Verification items for the finished model (mm, model axes). Face numbers are marked on the shaded views. A direction names the side the tool comes from. Round coordinates to 2 decimals unless told otherwise and drop trailing zeros. Order: outer loops, then holes, each group sorted by start corner. A loop starts at its lowest first (then second) coordinate and runs counter-clockwise, first axis right, second up. Notation, with made-up numbers: M -13,84.25 L 14,84.25 A35 ccw 14,119.25 Z; hole C -30,-21 d11. An arc over 180 degrees is marked long. Write item = value, one per line. Start each with the question number.
from build123d import *

# Parameters (mm, degrees)
SKETCH_1_W          = 35
SKETCH_1_H          = 53
EXTRUDE_1_DEPTH     = 2
SKETCH_2_W          = 2
SKETCH_2_H          = 53
EXTRUDE_2_DEPTH     = 13.2
SKETCH_3_W          = 31
SKETCH_3_H          = 3
EXTRUDE_3_DEPTH     = 7.2
SKETCH_4_W          = 31
SKETCH_4_H          = 3
EXTRUDE_4_DEPTH     = 13.2
CUT_EXTRUDE_1_REACH = 57.956
SKETCH_5_R          = 1.25
SKETCH_7_W          = 31
SKETCH_7_H          = 3
CUT_EXTRUDE_2_DEPTH = 2.2
SKETCH_8_W          = 31
SKETCH_8_H          = 3
CUT_EXTRUDE_3_DEPTH = 2
SKETCH_10_W         = 11
SKETCH_10_H         = 3
CUT_EXTRUDE_4_DEPTH = 4
CUT_EXTRUDE_START   = -3
SKETCH_9_R          = 1.25
CUT_EXTRUDE_5_DEPTH = 3
SKETCH_12_W         = 2
SKETCH_12_H         = 10
CUT_EXTRUDE_6_DEPTH = 4
SKETCH_13_W         = 33
SKETCH_13_H         = 47
CUT_EXTRUDE_7_DEPTH = 4


with BuildPart() as part:
    # 草图1 → 凸台-拉伸1 (new body)
    with BuildSketch(Plane.XY):
        with Locations((2.5, -6.5)):
            Rectangle(SKETCH_1_W, SKETCH_1_H)
    extrude(amount=EXTRUDE_1_DEPTH)

    # 草图2 → 凸台-拉伸2 (add)
    with BuildSketch(Plane.XY.offset(2)):
        with Locations((-14, -6.5)):
            Rectangle(SKETCH_2_W, SKETCH_2_H)
        with Locations((19, -6.5)):
            Rectangle(SKETCH_2_W, SKETCH_2_H)
    extrude(amount=EXTRUDE_2_DEPTH)

    # 草图3 → 凸台-拉伸3 (add)
    with BuildSketch(Plane.XY.offset(2)):
        with Locations((2.5, 18.5)):
            Rectangle(SKETCH_3_W, SKETCH_3_H)
        with Locations((2.5, -31.5)):
            Rectangle(SKETCH_3_W, SKETCH_3_H)
    extrude(amount=EXTRUDE_3_DEPTH)

    # 草图4 → 凸台-拉伸4 (add)
    with BuildSketch(Plane.XY.offset(2)):
        with Locations((2.5, 15.5)):
            Rectangle(SKETCH_4_W, SKETCH_4_H)
        with Locations((2.5, -28.5)):
            Rectangle(SKETCH_4_W, SKETCH_4_H)
    extrude(amount=EXTRUDE_4_DEPTH)

    # 草图5 → 切除-拉伸1 (cut, up to next)
    with BuildSketch(Plane(origin=(0, 17, 0), x_dir=(1, 0, 0), z_dir=(0, 1, 0)), mode=Mode.PRIVATE) as cut_extrude_1_sk1:
        with Locations(Location((-8, -11.2, 0), (0, 0, 270))):
            Circle(SKETCH_5_R)
    cut_extrude_1_tool1 = extrude(cut_extrude_1_sk1.sketch, amount=-CUT_EXTRUDE_1_REACH, mode=Mode.PRIVATE) & part.part
    # 草图5 → 切除-拉伸1 (cut, up to next)
    with BuildSketch(Plane(origin=(0, 17, 0), x_dir=(1, 0, 0), z_dir=(0, 1, 0)), mode=Mode.PRIVATE) as cut_extrude_1_sk2:
        with Locations(Location((2.5, -11.2, 0), (0, 0, 270))):
            Circle(SKETCH_5_R)
    cut_extrude_1_tool2 = extrude(cut_extrude_1_sk2.sketch, amount=-CUT_EXTRUDE_1_REACH, mode=Mode.PRIVATE) & part.part
    # 草图5 → 切除-拉伸1 (cut, up to next)
    with BuildSketch(Plane(origin=(0, 17, 0), x_dir=(1, 0, 0), z_dir=(0, 1, 0)), mode=Mode.PRIVATE) as cut_extrude_1_sk3:
        with Locations(Location((13, -11.2, 0), (0, 0, 270))):
            Circle(SKETCH_5_R)
    cut_extrude_1_tool3 = extrude(cut_extrude_1_sk3.sketch, amount=-CUT_EXTRUDE_1_REACH, mode=Mode.PRIVATE) & part.part
    add(cut_extrude_1_tool1.solids().sort_by_distance((-8, 17, 11.2))[0], mode=Mode.SUBTRACT)
    add(cut_extrude_1_tool2.solids().sort_by_distance((2.5, 17, 11.2))[0], mode=Mode.SUBTRACT)
    add(cut_extrude_1_tool3.solids().sort_by_distance((13, 17, 11.2))[0], mode=Mode.SUBTRACT)

    # 草图7 → 切除-拉伸2 (cut)
    with BuildSketch(Plane.XY.offset(15.2)):
        with Locations((2.5, 15.5)):
            Rectangle(SKETCH_7_W, SKETCH_7_H)
    extrude(amount=-CUT_EXTRUDE_2_DEPTH, mode=Mode.SUBTRACT)

    # 草图8 → 切除-拉伸3 (cut)
    with BuildSketch(Plane.XY.offset(15.2)):
        with Locations((2.5, -28.5)):
            Rectangle(SKETCH_8_W, SKETCH_8_H)
    extrude(amount=-CUT_EXTRUDE_3_DEPTH, mode=Mode.SUBTRACT)

    # 草图10 → 切除-拉伸4 (cut)
    with BuildSketch(Plane.XY.offset(13.2)):
        with Locations((2.5, -28.5)):
            Rectangle(SKETCH_10_W, SKETCH_10_H)
    extrude(amount=-CUT_EXTRUDE_4_DEPTH, mode=Mode.SUBTRACT)

    # 草图9 → 切除-拉伸5 (cut)
    with BuildSketch(Plane.XZ.offset(30).offset(CUT_EXTRUDE_START)):
        with Locations(Location((-8, 11.2, 0), (0, 0, 90))):
            Circle(SKETCH_9_R)
        with Locations(Location((13, 11.2, 0), (0, 0, 90))):
            Circle(SKETCH_9_R)
    extrude(amount=CUT_EXTRUDE_5_DEPTH, mode=Mode.SUBTRACT)

    # 草图12 → 切除-拉伸6 (cut)
    with BuildSketch(Plane.XY.offset(15.2)):
        with Locations((-14, -17.5)):
            Rectangle(SKETCH_12_W, SKETCH_12_H)
    extrude(amount=-CUT_EXTRUDE_6_DEPTH, mode=Mode.SUBTRACT)

    # 草图13 → 切除-拉伸7 (cut)
    with BuildSketch(Plane.XY.offset(2)):
        with Locations((2.5, -6.5)):
            Rectangle(SKETCH_13_W, SKETCH_13_H)
    extrude(amount=CUT_EXTRUDE_7_DEPTH, mode=Mode.SUBTRACT)


solid = part.part
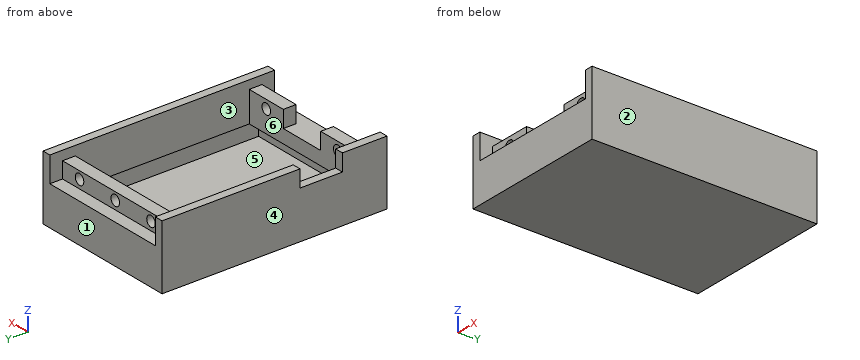
1) Cross-section at B-B, the plane x = -8. Enter the section's corners in (y, z), then the cut area to 3 significant figures.
2) Cross-section at A-A, the plane x = 2.5. Enter the section's corners in (y, z), then the cut area to 3 significant figures.
3) Access from +Z, -Z, +X, -X, +Y, -Y to the whole of each face (thin tool, end or side, straight path). Record for the marked faces 4, 5 and 6.
4) Scan lines: probe 1 along X at (y, z) = (15.2, 11.2); probe 2 along Z at (x, y) = (13, -28.65); probe 3 along Z at (x, y) = (17, 15.5). Record each from-to range of solid material in increasing order.
5) Release check for a two-part mould opening along Y. For the marked faces 1, 2 and 3 record: pulls with the +Y half, pulls with the -Y half, needs draft (parallel to the pull), parting line crosses it, or undercut.
6) Cross-section at D-D, the plane z = 7.75. Enter the section's corners in (x, y).
7) Gauge pin test, flat ends, axial feed: P1, Ø1.9, axis at x = 4.5, z = 10.5, coming from the +Y side; P2, Ø3, axis at x = -10, z = 12, coming from the -Y side; P3, Ø4, axis at x = -4, y = -19, coming from the +Z side. Record the tip position at first contact, or that the pin passes through.
8) Cross-section at C-C, the plane y = -18.5. Enter the section's corners in (x, z).
Geometry results:
q1.outline = M -33,0 L 20,0 L 20,9.2 L 17,9.2 L 17,9.95 L 14,9.95 L 14,6 L 17,6 L 17,2 L -30,2 L -30,6 L -27,6 L -27,9.95 L -30,9.95 L -30,9.2 L -33,9.2 Z; M -30,12.45 L -27,12.45 L -27,13.2 L -30,13.2 Z; M 14,12.45 L 17,12.45 L 17,13 L 14,13 Z
q1.area = 177 mm^2
q2.outline = M -33,0 L 20,0 L 20,9.2 L 17,9.2 L 17,9.95 L 14,9.95 L 14,6 L 17,6 L 17,2 L -30,2 L -30,6 L -27,6 L -27,9.2 L -33,9.2 Z; M 14,12.45 L 17,12.45 L 17,13 L 14,13 Z
q2.area = 172 mm^2
q3.face_4 = +Z, -Z, -X, +Y, -Y
q3.face_5 = none
q3.face_6 = +Z
q4.probe_1 = -15 to -9.25, -6.75 to 1.25, 3.75 to 11.75, 14.25 to 20
q4.probe_2 = 0 to 2, 6 to 9.95, 12.45 to 13.2
q4.probe_3 = 0 to 2, 6 to 13
q5.face_1 = pulls with the +Y half
q5.face_2 = needs draft
q5.face_3 = undercut
q6.outline = M -15,-33 L 20,-33 L 20,20 L -15,20 Z; hole M -13,-27 L 18,-27 L 18,14 L -13,14 Z
q7.P1 = 17
q7.P2 = -30
q7.P3 = 2
q8.outline = M -15,0 L 20,0 L 20,15.2 L 18,15.2 L 18,6 L 19,6 L 19,2 L -14,2 L -14,6 L -13,6 L -13,11.2 L -15,11.2 Z
